Autodesk Fusion 360 part; units mm, degrees
sketch "Sketch1" plane through (0, 0, 0) normal (1, 0, 0) x (0, 1, 0)
  line L0 (-75, -56.7965) -> (84.5885, -56.7965)
  line L1 (94.5885, -46.7965) -> (94.5885, 58.2035)
  line L2 (89.5885, 63.2035) -> (3.5272, 63.2035)
  line L3 (-70, 20.0323) -> (-2.9575, 20.0323)
  line L4 (-2.9575, 20.0323) -> (-1.469, 58.3973)
  line L5 (-97.4281, 59.7817) -> (-104.34, 62.6519) construction
  line L6 (-1.3367, 61.8082) -> (1.7233, 63.2035) construction
  line L7 (-85, 23.6607) -> (-92.9575, 20.0323) construction
  line L8 (-85, 51.039) -> (-85, 54.6209)
  line L9 (-85, 5.0323) -> (-85, -46.7965)
  line L10 (94.5885, -56.7965) -> (-33.3617, 20.0323) construction
  line L11 (-104.34, 62.6519) -> (-85, 51.039) construction
  line L12 (79.9542, 44.9695) -> (9.9542, 44.9695)
  line L13 (9.9542, 44.9695) -> (9.9542, 14.9695)
  line L14 (79.9542, 14.9695) -> (79.9542, 44.9695)
  line L15 (9.8967, -5.088) -> (59.8985, -5.088)
  line L16 (9.8971, 14.912) -> (9.8967, -5.088)
  line L17 (67.3, 44.9695) -> (94.5885, 63.2035) construction
  line L18 (79.9542, 14.9695) -> (59.8985, -5.088)
  line L19 (-85, -56.7965) -> (9.8969, 6.6131) construction
  line L20 (22.3522, 14.9356) -> (22.4384, 14.9932) construction
  line L21 (79.9542, 44.9695) -> (9.8971, 44.9695)
  line L22 (9.8971, 44.9695) -> (9.8971, 14.912)
  line L23 (9.8971, 14.912) -> (79.9542, 14.912)
  line L24 (79.9542, 14.912) -> (79.9542, 44.9695)
  line L25 (9.9542, 14.9695) -> (59.8985, 14.9695)
  line L26 (59.8985, 14.9695) -> (59.8985, -5.088)
  line L27 (59.8985, -5.088) -> (9.9542, -5.088)
  line L28 (9.9542, -5.088) -> (9.9542, 14.9695)
  arc A0 (-70, 20.0323) -> (-85, 5.0323) centre (-70, 5.0323) ccw
  arc A1 (84.5885, -56.7965) -> (94.5885, -46.7965) centre (84.5885, -46.7965) ccw
  arc A2 (-85, -46.7965) -> (-75, -56.7965) centre (-75, -46.7965) ccw
  arc A3 (94.5885, 58.2035) -> (89.5885, 63.2035) centre (89.5885, 58.2035) ccw
  arc A4 (3.5272, 63.2035) -> (-1.469, 58.3973) centre (3.5272, 58.2035) ccw
  line L29 (79.9542, 44.9695) -> (9.9542, 44.9695)
  line L30 (9.9542, 44.9695) -> (9.9542, 54.9695)
  line L31 (9.9542, 54.9695) -> (79.9542, 54.9695)
  line L32 (79.9542, 54.9695) -> (79.9542, 44.9695)
  line L33 (74.9542, -19.6144) -> (14.9542, -19.6144)
  line L34 (9.9542, -24.6144) -> (9.9542, -46.6144)
  line L35 (14.9542, -51.6144) -> (74.9542, -51.6144)
  line L36 (79.9542, -46.6144) -> (79.9542, -24.6144)
  arc A5 (14.9542, -19.6144) -> (9.9542, -24.6144) centre (14.9542, -24.6144) ccw
  arc A6 (9.9542, -46.6144) -> (14.9542, -51.6144) centre (14.9542, -46.6144) ccw
  arc A7 (79.9542, -24.6144) -> (74.9542, -19.6144) centre (74.9542, -24.6144) ccw
  arc A8 (74.9542, -51.6144) -> (79.9542, -46.6144) centre (74.9542, -46.6144) ccw
  point P0 (79.9542, -19.6144)
  point P1 (9.9542, -19.6144)
  point P2 (79.9542, -51.6144)
  dimension "d1" = 180
  dimension "d2" = 120
  dimension "d3" = 90
  dimension "d4" = 40
  dimension "d5" = 70
  dimension "d6" = 30
  dimension "d10" = 15
  dimension "d11" = 10
  dimension "d12" = 10
  dimension "d13" = 5
  dimension "d14" = 5
  dimension "d15" = 70
  dimension "d16" = 10
  dimension "d17" = 70
  dimension "d18" = 32
  dimension "d19" = 5
  dimension "d20" = 5
  dimension "d21" = 5
  dimension "d22" = 5
extrude "Extrude1" add sketch "Sketch1" along normal blind 150
sketch "Sketch2" plane through (0, 0, 0) normal (0, 1, 0) x (1, 0, 0)
  line L0 (15.2809, -58.615) -> (135.2809, -58.615)
Work out the finished part from the listing and answer in its coordinate system (mm). A direction names the side the tool comes from. Coordinates: 2 decimals unless noted, no trailing zeros. Order: outer loops, then holes, each group sorted by start corner. A loop starts at its lowest first (then second) coordinate and runs counter-clockwise, first axis right, second up. Notation, with made-up numbers: (-37, -10.75) - (6, -10.75) arc R35 cw to (6, 25.25) - close; hole circle Ø1 at (18, -37.75). An arc over 180 degrees is marked (long way). Put each result on its own line as item: value. Start each with the question number.
1) Find section C-C (z = 12.5). Give the vertices of the cut face in (x, y).
2) Find section B-B (x = 110.5). Give the vertices of the cut face in (y, z), plus the area to 3 significant figures.
3) For a pull along Y with two mould halves and no side action, classify faces 4 (the flat face through (74, 9.954, -35)), 5 (the flat face through (74, 47, 63.204)), 6 (the cylindrical face through (73.95, 0.022, 61.77)) as released by +Y, released by -Y, zero draft, split by the parting line, or undercut.
4) A flat-ended cylindrical pin translates along its axis: pin 1 (12 mm diameter, centred on x = 106.5, z = 40, fed in from -Y). Find the tip coordinate at first contact, or state that the pin passes through.
5) For faces 1 (the flat face through (74, 35, -5.088)), 2 (the flat face through (0, 4, -9)), 3 (the flat face through (74, -37, 20.032)), determine the directions among +Z, -Z, +X, -X, +Y, -Y from which every point of the face is accessible in a straight line to the end or side of a thin tool.
6) Find section D-D (z = 48.5). Give the vertices of the cut face in (x, y).
7) Find section A-A (y = 46). Give the vertices of the cut face in (x, z).
8) Find the intervals of material crossed by line 1 (Z direction, x = 91.5, y = 19); line 2 (Y direction, x = 33.5, z = -42); line 3 (Z direction, x = 142, y = 73), in increasing order. Write a range as from..to.
Results list:
1. outline: (0, -83.01) - (150, -83.01) - (150, 9.9) - (0, 9.9) - close; (0, 77.48) - (150, 77.48) - (150, 94.59) - (0, 94.59) - close
2. outline: (-85, -46.8) arc R10 ccw to (-75, -56.8) - (84.59, -56.8) arc R10 ccw to (94.59, -46.8) - (94.59, 58.2) arc R5 ccw to (89.59, 63.2) - (3.53, 63.2) arc R5 ccw to (-1.47, 58.4) - (-2.96, 20.03) - (-70, 20.03) arc R15 ccw to (-85, 5.03) - close; hole (9.9, -5.09) - (59.9, -5.09) - (79.9, 14.91) - (79.95, 14.91) - (79.95, 54.97) - (9.95, 54.97) - (9.95, 44.97) - (9.9, 44.97) - (9.9, 14.91) - close; hole (9.95, -46.61) arc R5 ccw to (14.95, -51.61) - (74.95, -51.61) arc R5 ccw to (79.95, -46.61) - (79.95, -24.61) arc R5 ccw to (74.95, -19.61) - (14.95, -19.61) arc R5 ccw to (9.95, -24.61) - close
2. area: 11,600 mm^2
3. face 4: undercut
3. face 5: zero draft
3. face 6: released by -Y
4. pin 1: stops at y = -2.42
5. face 1: +X, -X
5. face 2: +Z, -Z, -X, +Y, -Y
5. face 3: +Z, +X, -X, -Y
6. outline: (0, -1.85) - (150, -1.85) - (150, 9.95) - (0, 9.95) - close; (0, 79.95) - (150, 79.95) - (150, 94.59) - (0, 94.59) - close
7. outline: (0, -56.8) - (150, -56.8) - (150, -51.61) - (0, -51.61) - close; (0, -19.61) - (150, -19.61) - (150, -5.09) - (0, -5.09) - close; (0, 54.97) - (150, 54.97) - (150, 63.2) - (0, 63.2) - close
8. line 1: z = -56.8..-51.61, -19.61..-5.09, 54.97..63.2
8. line 2: y = -85..9.95, 79.95..94.59
8. line 3: z = -56.8..-51.61, -19.61..8.01, 54.97..63.2
